Read the model definition and answer for the solid it produces. Units are mm, in the model's axes. Coordinates: 2 decimals unless noted, no trailing zeros. Write each loop counter-clockwise with the first axis right and the second up, starting at its lowest first coordinate (ties: lowest second). Pieces come first, ordered by that corner, then holes. Notation, with made-up numbers: M -7,-34 L 25,-34 A18 ccw 25,-28 Z; hole C 66.5,76 d6. An arc over 180 degrees is marked long. Write item = value, one per line.
from build123d import *

# Parameters (mm, degrees)
SKETCH1_W           = 393.7
SKETCH1_H           = 393.7
BOSS_EXTRUDE1_DEPTH = 3.175
SKETCH2_W           = 342.9
SKETCH2_H           = 342.9
CUT_EXTRUDE1_DEPTH  = 279.40604452
SKETCH3_R           = 1.905
SKETCH3_R_2         = 2.01965575
CUT_EXTRUDE2_DEPTH  = 279.40604452


with BuildPart() as part:
    # Sketch1 → Boss-Extrude1 (new body)
    with BuildSketch(Plane(origin=(0, 0, 0), x_dir=(1, 0, 0), z_dir=(0, 1, 0))):
        Rectangle(SKETCH1_W, SKETCH1_H)
    extrude(amount=BOSS_EXTRUDE1_DEPTH)

    # Sketch2 → Cut-Extrude1 (cut, through all)
    with BuildSketch(Plane(origin=(0, 3.175, 0), x_dir=(1, 0, 0), z_dir=(0, 1, 0))):
        Rectangle(SKETCH2_W, SKETCH2_H)
    extrude(amount=-CUT_EXTRUDE1_DEPTH, mode=Mode.SUBTRACT)

    # Sketch3 → Cut-Extrude2 (cut, through all)
    with BuildSketch(Plane(origin=(0, 3.175, 0), x_dir=(1, 0, 0), z_dir=(0, 1, 0))):
        with Locations(Location((-104.775, -193.675, 0), (0, 0, 270))):
            Circle(SKETCH3_R)
        with Locations(Location((104.775, -193.675, 0), (0, 0, 270))):
            Circle(SKETCH3_R)
        with Locations(Location((-193.675, -104.775, 0), (0, 0, 270))):
            Circle(SKETCH3_R)
        with Locations(Location((-193.675, 104.775, 0), (0, 0, 270))):
            Circle(SKETCH3_R)
        with Locations(Location((-104.775, 193.675, 0), (0, 0, 270))):
            Circle(SKETCH3_R)
        with Locations(Location((104.775, 193.675, 0), (0, 0, 270))):
            Circle(SKETCH3_R_2)
        with Locations(Location((193.675, 104.775, 0), (0, 0, 270))):
            Circle(SKETCH3_R)
        with Locations(Location((193.675, -104.775, 0), (0, 0, 270))):
            Circle(SKETCH3_R)
    extrude(amount=-CUT_EXTRUDE2_DEPTH, mode=Mode.SUBTRACT)


solid = part.part
Item 1: Consider line 1 along X through (y, z) = (1.1, 25.5); line 2 along Z through (x, y) = (-103.5, 2.8). Determine where each line is inside the solid, lowest interval first. Write a range as from..to.
Worked answers:
line_1 = -196.85..-171.45, 171.45..196.85
line_2 = -196.85..-195.09, -192.26..-171.45, 171.45..192.26, 195.09..196.85
Item 2: Find section A-A (z = 39.5). Determine the outline of the cut face in (x, y) (3 decimals).
Worked answers:
outline = M -196.85,0 L -171.45,0 L -171.45,3.175 L -196.85,3.175 Z; M 171.45,0 L 196.85,0 L 196.85,3.175 L 171.45,3.175 Z
Item 3: Find section C-C (y = 2.15). State how many separate pieces and enclosed holes the cut face has, and give its area (3 significant figures).
Worked answers:
separate_pieces = 1
enclosed_holes = 9
area = 37,300 mm²
Item 4: Find section B-B (x = 43.5). Determine the outline of the cut face in (y, z) (3 decimals).
Worked answers:
outline = M 0,-196.85 L 3.175,-196.85 L 3.175,-171.45 L 0,-171.45 Z; M 0,171.45 L 3.175,171.45 L 3.175,196.85 L 0,196.85 Z
